Design review of the part shown in the three views and the two pictorial views. Dimensions are in mm from the part's minimum x, y and z. A direction names the side the tool comes from. Coordinates: 2 decimals unless noted, no trailing zeros. Write each loop counter-clockwise with the first axis right and the second up, starting at its lowest first coordinate (ties: lowest second). Pieces come first, ordered by that corner, then holes. Notation, with made-up numbers: (26, -30) - (66, -30) arc R22 ccw to (66, 9) - close; hole circle Ø4 at (62.25, 51.5). An arc over 180 degrees is marked (long way). Answer as CSV lines item,"result". Start each with the question number.
Q1. For line 1 along X through (y, z) = (17, 5.5); line 2 along X through (y, z) = (14, 5.5); line 3 along Y through (x, z) = (9.25, 2.25), list the stretches that pass through material, from the lowest coordinate up. Write a range as [from, to].
Q2. We need section C-C (z = 5.5). Write out the cut boundary in (x, y), plus the area to 3 significant figures.
Q3. Mouldability with a two-part tool opening along X and no side actions: class the marked faces 1, 2 and 3 as pulls with the +X half, pulls with the -X half, needs draft (parallel to the pull), parting line crosses it, or undercut.
Q4. Clearance check with flat-ended pins moving along their axes: pin 1 (2.5 mm diameter, centred on y = 3.5, z = 6, fed in from -X); pin 2 (3.5 mm diameter, centred on x = 5.5, y = 4, fed in from +Z); pin 3 (5.5 mm diameter, centred on x = 5.5, z = 5.5, fed in from -Y). State where each tip first meets the part, or that it passes through.
Q5. Machinability: for the marked faces 4, 5 and 6, which of the approach directions +Z, -Z, +X, -X, +Y, -Y give a long, thin tool a straight path to every point of the face, cutting with its end or side? Answer none if there is none.
Q6. We need section A-A (y = 13). Write out the cut boundary in (x, z), plus the area to 3 significant figures.
Q7. We need section B-B (x = 5.5). Write out the cut boundary in (y, z), plus the area to 3 significant figures.
Q8. We need section D-D (y = 9). Write out the cut boundary in (x, z).
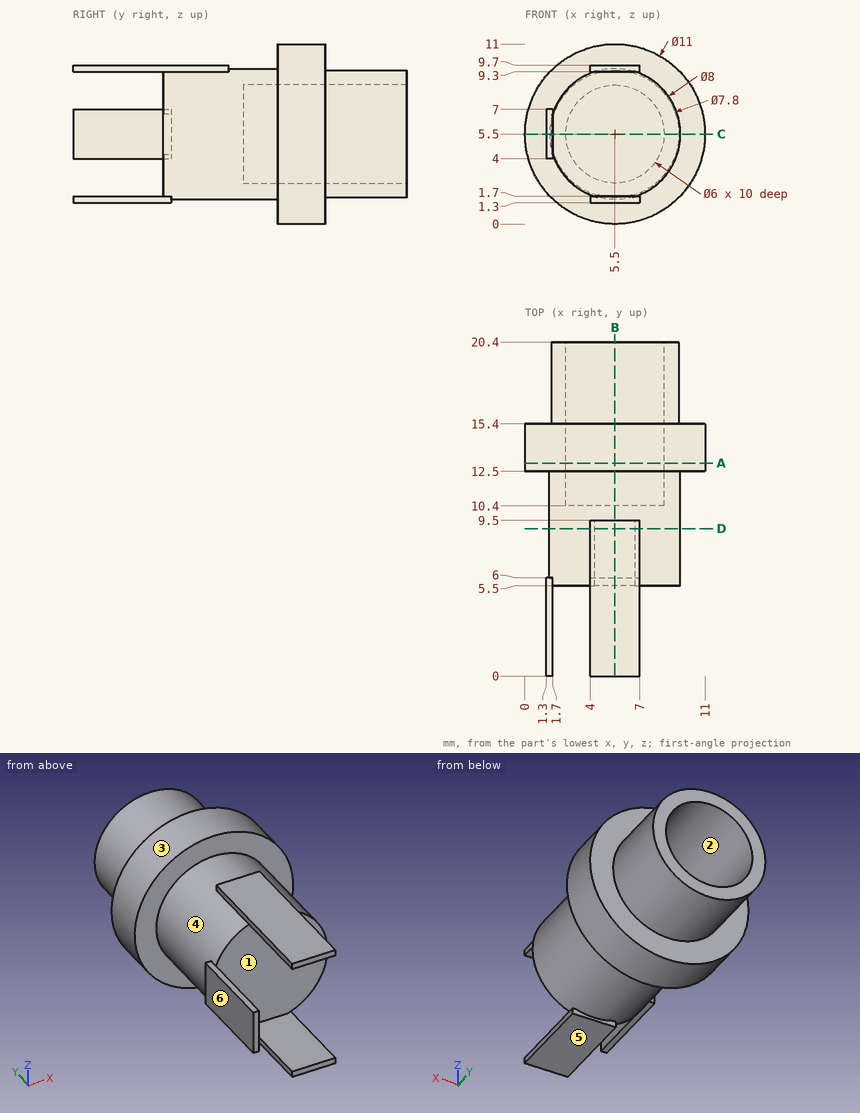
Results list:
1,line 1,"x = [1.6, 2.5], [8.5, 9.4]"
1,line 2,"x = [0, 2.5], [8.5, 11]"
1,line 3,"y = [12.5, 15.4]"
2,outline,"(0, 12.5) - (1.5, 12.5) - (1.5, 6) - (1.3, 6) - (1.3, 0) - (1.7, 0) - (1.7, 5.5) - (9.5, 5.5) - (9.5, 12.5) - (11, 12.5) - (11, 15.4) - (9.4, 15.4) - (9.4, 20.4) - (8.5, 20.4) - (8.5, 10.4) - (2.5, 10.4) - (2.5, 20.4) - (1.6, 20.4) - (1.6, 15.4) - (0, 15.4) - close"
2,area,"69.2 mm2"
3,face 1,"needs draft"
3,face 2,"undercut"
3,face 3,"parting line crosses it"
4,pin 1,"stops at x = 1.3"
4,pin 2,"stops at z = 9.7"
4,pin 3,"stops at y = 5.5"
5,face 4,"none"
5,face 5,"-Z, +X, -X, -Y"
5,face 6,"+Z, -Z, -X, -Y"
6,outline,"circle Ø11 at (5.5, 5.5); hole circle Ø6 at (5.5, 5.5)"
6,area,"66.8 mm2"
7,outline,"(0, 1.3) - (6, 1.3) - (6, 1.5) - (12.5, 1.5) - (12.5, 0) - (15.4, 0) - (15.4, 1.6) - (20.4, 1.6) - (20.4, 2.5) - (10.4, 2.5) - (10.4, 8.5) - (20.4, 8.5) - (20.4, 9.4) - (15.4, 9.4) - (15.4, 11) - (12.5, 11) - (12.5, 9.5) - (9.5, 9.5) - (9.5, 9.7) - (0, 9.7) - (0, 9.3) - (5.5, 9.3) - (5.5, 1.7) - (0, 1.7) - close"
7,area,"72.2 mm2"
8,outline,"(4, 9.3) - (4.25, 9.3) arc R4 ccw (long way) to (6.75, 9.3) - (7, 9.3) - (7, 9.7) - (4, 9.7) - close"
